Autodesk Inventor part; units mm, degrees
ref_plane "YZ Plane" through (0, 0, 0) normal (1, 0, 0) x (0, 1, 0)
ref_plane "XZ Plane" through (0, 0, 0) normal (0, 1, 0) x (-1, 0, 0)
ref_plane "XY Plane" through (0, 0, 0) normal (0, 0, 1) x (1, 0, 0)
sketch "Skizze1" plane through (0, 0, 0) normal (0, 1, 0) x (-1, 0, 0)
  line L0 (87.5, -100) -> (-87.5, -100)
  line L1 (-87.5, -100) -> (-87.5, 100)
  line L2 (-87.5, 100) -> (87.5, 100)
  line L3 (87.5, 100) -> (87.5, -100)
  line L4 (0, -140) -> (0, 140)
  line L5 (-122.5, 0) -> (122.5, 0)
  point P0 (0, 0)
  dimension "d0" = 175
  dimension "d1" = 200
extrude "Extrusion1" add sketch "Skizze1" along normal blind 2
sketch "Skizze2" plane through (0, 2, 0) normal (0, 1, 0) x (1, 0, 0)
  circle A0 centre (-54.5, 95) radius 1.6
  line L0 (0, 140) -> (0, -140)
  line L1 (122.5, 0) -> (-122.5, 0)
  line L2 (87.5, 100) -> (-87.5, 100)
  circle A1 centre (82.5, 95) radius 1.6
  circle A2 centre (-54.5, -95) radius 1.6
  circle A3 centre (82.5, -95) radius 1.6
  line L3 (-87.5, 100) -> (-87.5, -100)
  line L4 (87.5, -100) -> (87.5, 100)
  point P0 (0, 0)
  dimension "d4" = 3.2
  dimension "d6" = 5
  dimension "d7" = 3.2
  dimension "d9" = 5
  dimension "d40" = 33
  dimension "d41" = 5
extrude "Extrusion2" cut sketch "Skizze2" against normal up to surface (2 mm away) contours A0 | A1 | A2 | A3
sketch "Skizze3" plane through (0, 2, 0) normal (0, 1, 0) x (1, 0, 0)
  line L0 (87.5, -100) -> (87.5, 100)
  line L1 (-87.5, -100) -> (87.5, -100)
  line L2 (87.5, 100) -> (-87.5, 100)
  circle A0 centre (-64.5, 89.5) radius 1.6
  line L3 (-87.5, 100) -> (-87.5, -100)
  circle A1 centre (-64.5, 25.5) radius 1.6
  circle A2 centre (-64.5, -25.5) radius 1.6
  circle A3 centre (-64.5, -89.5) radius 1.6
  point P0 (0, 0)
  dimension "d26" = 3.2
  dimension "d27" = 23
  dimension "d28" = 10.5
  dimension "d29" = 3.2
  dimension "d30" = 23
  dimension "d31" = 74.5
  dimension "d32" = 3.2
  dimension "d33" = 23
  dimension "d34" = 74.5
  dimension "d35" = 3.2
  dimension "d36" = 10.5
  dimension "d37" = 23
extrude "Extrusion4" cut sketch "Skizze3" against normal up to surface (2 mm away) contours A0 | A1 | A2 | A3
sketch "Skizze4" plane through (0, 2, 0) normal (0, 1, 0) x (1, 0, 0)
  line L0 (-82.5, -12) -> (-72.5, -12)
  line L1 (-72.5, -12) -> (-72.5, 12)
  line L2 (-72.5, 12) -> (-82.5, 12)
  line L3 (-82.5, 12) -> (-82.5, -12)
  line L4 (-82.5, -12) -> (-72.5, 12) construction
  line L5 (-72.5, -12) -> (-82.5, 12) construction
  line L6 (-87.5, 100) -> (-87.5, -100)
  line L7 (87.5, 100) -> (-87.5, 100)
  point P0 (0, 0)
  point P1 (-77.5, 0)
  dimension "d42" = 10
  dimension "d43" = 24
  dimension "d44" = 5
  dimension "d45" = 88
extrude "Extrusion5" cut sketch "Skizze4" against normal up to surface (2 mm away)
fillet "Rundung1" radius 2 1 edges at (-82.5, 0, 0)
fillet "Rundung2" radius 2 1 edges at (-72.5, 2, 0)
sketch "Skizze5" plane through (0, 2, 0) normal (0, 1, 0) x (1, 0, 0)
  circle A0 centre (-32.5, 76.5) radius 3.5
  circle A1 centre (33.5, 76.5) radius 3.5
  circle A2 centre (-32.5, 50.5) radius 3.5
  circle A3 centre (33.5, 50.5) radius 3.5
  line L0 (87.5, 100) -> (-87.5, 100)
  line L1 (-87.5, 100) -> (-87.5, -100)
  line L2 (45.5, 85) -> (78.5, 85)
  line L3 (78.5, 85) -> (78.5, 30)
  line L4 (78.5, 30) -> (45.5, 30)
  line L5 (45.5, 30) -> (45.5, 85)
  line L6 (122.5, 0) -> (-122.5, 0)
  circle A4 centre (-32.5, -76.5) radius 3.5
  circle A5 centre (33.5, -76.5) radius 3.5
  circle A6 centre (-32.5, -50.5) radius 3.5
  circle A7 centre (33.5, -50.5) radius 3.5
  line L7 (45.5, -85) -> (78.5, -85)
  line L8 (78.5, -85) -> (78.5, -30)
  line L9 (78.5, -30) -> (45.5, -30)
  line L10 (45.5, -30) -> (45.5, -85)
  circle A8 centre (-52.5, 23) radius 3.5
  circle A9 centre (-52.5, -23) radius 3.5
  circle A10 centre (13.5, 23) radius 3.5
  circle A11 centre (13.5, -23) radius 3.5
  line L11 (53.5, 15) -> (78.5, 15)
  line L12 (78.5, 15) -> (78.5, -15)
  line L13 (78.5, -15) -> (53.5, -15)
  line L14 (53.5, -15) -> (53.5, 15)
  line L15 (87.5, -100) -> (87.5, 100)
  point P0 (0, 0)
  dimension "d50" = 7
  dimension "d51" = 7
  dimension "d52" = 7
  dimension "d53" = 7
  dimension "d54" = 23.5
  dimension "d55" = 23.5
  dimension "d56" = 55
  dimension "d57" = 66
  dimension "d58" = 55
  dimension "d59" = 66
  dimension "d60" = 26
  dimension "d61" = 26
  dimension "d62" = 33
  dimension "d63" = 12
  dimension "d64" = 15
  dimension "d65" = 55
  dimension "d81" = 7
  dimension "d82" = 7
  dimension "d83" = 7
  dimension "d84" = 7
  dimension "d85" = 35
  dimension "d86" = 35
  dimension "d87" = 46
  dimension "d88" = 46
  dimension "d89" = 23
  dimension "d90" = 23
  dimension "d91" = 66
  dimension "d92" = 66
  dimension "d93" = 25
  dimension "d94" = 30
  dimension "d95" = 9
extrude "Extrusion6" add sketch "Skizze5" along normal blind 7 contours A0 | A1 | A2 | A3 | A4 | A5 | A6 | A7
extrude "Extrusion8" cut sketch "Skizze5" against normal up to surface (2 mm away) contours L12 L13 L14 L6 | L6 L14 L11 L12 | L2 L3 L4 L5 | L10 L9 L8 L7
fillet "Rundung3" radius 2 3 edges at (45.5, 2, -57.5) (45.5, 2, 57.5) (53.5, 2, 0)
extrude "Extrusion9" add sketch "Skizze5" along normal blind 18 contours A8 | A9 | A10 | A11
sketch "Skizze6" plane through (-32.5, 9, -76.5) normal (0, 1, 0) x (1, 0, 0)
  circle A0 centre (0, 0) radius 3.5
  circle A1 centre (0, -26) radius 3.5
  circle A2 centre (66, -26) radius 3.5
  circle A3 centre (66, 0) radius 3.5
  circle A4 centre (66, -127) radius 3.5
  circle A5 centre (66, -153) radius 3.5
  circle A6 centre (0, -153) radius 3.5
  circle A7 centre (0, -127) radius 3.5
  circle A8 centre (0, 0) radius 2
  circle A9 centre (0, -26) radius 2
  circle A10 centre (66, -26) radius 2
  circle A11 centre (66, 0) radius 2
  circle A12 centre (0, -127) radius 3.5
  circle A13 centre (0, -127) radius 2
  circle A14 centre (0, -153) radius 2
  circle A15 centre (66, -127) radius 3.5
  circle A16 centre (66, -127) radius 2
  circle A17 centre (66, -153) radius 2
  point P0 (32.5, -76.5)
  dimension "d68" = 4
  dimension "d69" = 4
  dimension "d70" = 4
  dimension "d71" = 4
  dimension "d72" = 4
  dimension "d73" = 4
  dimension "d74" = 4
  dimension "d75" = 4
extrude "Extrusion7" cut sketch "Skizze6" against normal blind 5 contours A8 | A9 | A10 | A11 | A13 | A14 | A16 | A17
sketch "Skizze8" plane through (-52.5, 20, -23) normal (0, 1, 0) x (1, 0, 0)
  circle A0 centre (0, 0) radius 3.5
  circle A1 centre (66, 0) radius 3.5
  circle A2 centre (66, -46) radius 3.5
  circle A3 centre (0, -46) radius 3.5
  circle A4 centre (0, 0) radius 3.5
  circle A5 centre (0, 0) radius 2
  circle A6 centre (66, 0) radius 3.5
  circle A7 centre (66, 0) radius 2
  circle A8 centre (66, -46) radius 3.5
  circle A9 centre (66, -46) radius 2
  circle A10 centre (0, -46) radius 3.5
  circle A11 centre (0, -46) radius 2
  point P0 (52.5, -23)
  dimension "d98" = 4
  dimension "d99" = 4
  dimension "d100" = 4
  dimension "d101" = 4
extrude "Extrusion10" cut sketch "Skizze8" against normal blind 5 contours A5 | A7 | A9 | A11
sketch "Skizze9" plane through (0, 2, 0) normal (0, 1, 0) x (1, 0, 0)
  circle A0 centre (-52.5, 22.75) radius 1.75
  circle A1 centre (-32.5, 51.5) radius 1
  line L0 (-52.5, 22.75) -> (-32.5, 51.5)
  circle A2 centre (-47.354, 30.1473) radius 1.6
  circle A3 centre (-37.646, 44.1027) radius 1.6
  circle A4 centre (-42.5, 37.125) radius 0.1
  circle A5 centre (-72.5, 55) radius 1.6
  circle A6 centre (-72.5, 38) radius 1.6
  line L1 (-87.5, 100) -> (-87.5, -100)
  line L2 (122.5, 0) -> (-122.5, 0)
  line L3 (87.5, 100) -> (-87.5, 100)
  circle A7 centre (-32.5, 50.5) radius 3.5
  circle A8 centre (-52.5, 23) radius 3.5
  point P0 (0, 0)
  dimension "d104" = 3.2
  dimension "d105" = 3.2
  dimension "d106" = 13.8
  dimension "d107" = 0.2
  dimension "d108" = 6.8
  dimension "d109" = 3.2
  dimension "d110" = 3.2
  dimension "d111" = 15
  dimension "d112" = 15
  dimension "d113" = 17
  dimension "d134" = 55.8973
  dimension "d135" = 49.8541
  dimension "d136" = 40.1459
  dimension "d137" = 45
  dimension "d138" = 1.5
  dimension "d139" = 1.5
extrude "Extrusion11" cut sketch "Skizze9" against normal up to surface (2 mm away) contours A3 L0 | L0 A3 | A2 L0 | L0 A2 | A5 | A6
sketch "Skizze10" plane through (0, 2, 0) normal (0, 1, 0) x (1, 0, 0)
  line L0 (-1, -90.8) -> (6, -90.8)
  line L1 (6, -90.8) -> (6, -97.8)
  line L2 (6, -97.8) -> (-1, -97.8)
  line L3 (-1, -97.8) -> (-1, -90.8)
  line L4 (-87.5, -100) -> (87.5, -100)
  line L5 (87.5, -100) -> (87.5, 100)
  line L6 (122.5, 0) -> (-122.5, 0)
  line L7 (-1, 90.8) -> (6, 90.8)
  line L8 (6, 90.8) -> (6, 97.8)
  line L9 (6, 97.8) -> (-1, 97.8)
  line L10 (-1, 97.8) -> (-1, 90.8)
  point P0 (0, 0)
  dimension "d117" = 7
  dimension "d118" = 7
  dimension "d119" = 2.2
  dimension "d120" = 81.5
extrude "Extrusion12" add sketch "Skizze10" along normal blind 9
sketch "Skizze11" plane through (-1, 2, 97.8) normal (0, 0, 1) x (1, 0, 0)
  circle A0 centre (3.5, 5) radius 2
  line L0 (7, 0) -> (0, 0)
  line L1 (7, 0) -> (7, 9)
  point P0 (1, -2)
  dimension "d123" = 4
  dimension "d124" = 5
  dimension "d125" = 3.5
extrude "Extrusion13" cut sketch "Skizze11" against normal blind 5
sketch "Skizze12" plane through (6, 2, -97.8) normal (0, 0, -1) x (-1, 0, 0)
  circle A0 centre (3.5, 5) radius 2
  line L0 (7, 0) -> (0, 0)
  line L1 (7, 0) -> (7, 9)
  point P0 (6, -2)
  dimension "d128" = 4
  dimension "d129" = 5
  dimension "d130" = 3.5
extrude "Extrusion14" cut sketch "Skizze12" against normal blind 5
fillet "Rundung4" radius 3.5 4 edges at (6, 11, -94.3) (-1, 11, -94.3) (-1, 11, 94.3) (6, 11, 94.3)
properties part number "_3D-Druck"
Geometry: final body of the model. Coordinates: model frame, mm. A direction names the side the tool comes from. Give positions to 0.01 mm unless a question says otherwise; leave off trailing zeros. Loops run counter-clockwise (first coordinate to the right, second up) from the corner with the lowest first, then second, coordinate; pieces in that order, holes last. Notation, with made-up numbers: (36, 47) -> (75, 47) arc R24 cw to (75, 74) -> close; hole circle Ø7 at (-30.5, 45). An arc over 180 degrees is marked (long way). Use one line per item in the form item = value.
Item 1: Access query for faces 1 (the face through (3, 7, -92.8)), 2 (the face through (-1, 5, -94)), 3 (the face through (3, 4, -97.8)), 4 (the face through (-33, 4, 76)). Directions: +Z, -Z, +X, -X, +Y, -Y. A direction counts if a zero-diameter tool reaches every point of the face in a straight line with its end or side. Return the directions, or none.
A:
face_1 = -Z
face_2 = +Z, -Z, -X, +Y
face_3 = -Z, +X, -X, +Y
face_4 = +Y
Item 2: Line query: probe 1 along Z at (x, y) = (-72.5, 1.15); probe 2 along Z at (x, y) = (-52.5, 17.5); probe 3 along Z at (x, y) = (-64.5, 1.15). Output: solid intervals per line, ascending.
A:
probe_1 = -100 to -56.6, -53.4 to -39.6, -36.4 to -12, 12 to 100
probe_2 = -26.5 to -25, -21 to -19.5, 19.5 to 21, 25 to 26.5
probe_3 = -100 to -91.1, -87.9 to -27.1, -23.9 to 23.9, 27.1 to 87.9, 91.1 to 100
Item 3: Pin query (flat end, axial travel): P1, Ø2, axis at x = 15, y = 12, coming from the -Z side; P2, Ø5, axis at x = 82.5, z = 95, coming from the +Y side; P3, Ø6, axis at y = 5.5, z = -94, coming from the -X side. Return the tip coordinate at first contact, or that it passes through.
A:
P1 = -26.46
P2 = 2
P3 = -1
Item 4: Draft query along Y for faces 5 (the face through (-53, 15, 23)), 6 (the face through (2.24, 8.983, 95.335)), 7 (the face through (-56, 11, -23)). Return one class per face: pulls with the +Y half, pulls with the -Y half, needs draft (parallel to the pull), parting line crosses it, or undercut.
A:
face_5 = pulls with the +Y half
face_6 = undercut
face_7 = needs draft
Item 5: Section query B-B on x = -21.5. Output: boundary loops of the cut face in (y, z), and give its area (3 significant figures).
A:
outline = (0, -100) -> (2, -100) -> (2, 100) -> (0, 100) -> close
area = 400 mm^2
